Work out the finished part from the listing and answer in its coordinate system (mm). A direction names the side the tool comes from. Coordinates: 2 decimals unless noted, no trailing zeros. Order: outer loops, then holes, each group sorted by start corner. A loop starts at its lowest first (then second) coordinate and runs counter-clockwise, first axis right, second up. Notation, with made-up numbers: M 22,3 L 66,3 A16 cw 66,15 Z; hole C -11.5,38 d9. An arc over 180 degrees is marked long. Answer in a Markdown table with one row per item. Add a question column.
Item 1: Flat-ended cylindrical pins translate along their axes: pin 1 Ø3 at (x, z) = (1.5, 7) entering from -Y; pin 2 Ø1.1 at (x, y) = (2, 5) entering from +Z; pin 3 Ø5 at (x, z) = (-1, 112) entering from +Y; pin 4 Ø3 at (x, y) = (-3, 0) entering from -Z. Find the tip coordinate at first contact, or state that the pin passes through.
Item 2: Consider line 1 (X direction, y = 0, z = 7) (3 decimals); line 2 (Y direction, x = 0, z = 7.5) (3 decimals); line 3 (Y direction, x = 0.5, z = 112). Determine where each line is inside the solid, lowest interval first. Write a range as from..to.
Item 3: The part is cut by section D-D (z = 37). Write down the section's boundary in (x, y), then the cut area to 3 significant figures.
Item 4: The mould has two halves that part along X. Classify faces 5 (the face through (-1.38, -6.2, 62.61)), 6 (the face through (-2, 3, 0)), 7 (the face through (0, 0, 13.335)): released by +X, released by -X, zero draft, split by the parting line, or undercut.
Item 5: The part is cut by section A-A (y = 0). Write down the section's boundary in (x, z) (3 decimals), then the cut area to 3 significant figures.
Item 6: The part is cut by section B-B (x = 0). Write down the section's boundary in (y, z) (3 decimals).
Item 7: Which of the six approach directions +Z, -Z, +X, -X, +Y, -Y give full straight-line access (tool end or side, diameter ignored) to faces 1 (the face through (0, 5, 25.4)), 2 (the face through (-0.69, 3.1, 6.57)), 3 (the face through (0, -5, 25.4)), 4 (the face through (0, 4.191, 114))?
Item 8: The part is cut by section C-C (z = 19.5). Write down the section's boundary in (x, y), then the cut area to 3 significant figures.
from build123d import *

# Parameters (mm, degrees)
F0_R     = 6.35
F1_DEPTH = 127
F2_R     = 3.175
F3_DEPTH = 13.335
F4_R     = 3.175
F5_DEPTH = 13.335
F7_DEPTH = 25.4
F9_DEPTH = 25.4


with BuildPart() as f1:
    # F0 (on Top) → F1 (new body)
    with BuildSketch(Plane.XY):
        Circle(F0_R)
    extrude(amount=F1_DEPTH)

    # F2 (on face) → F3 (cut)
    with BuildSketch(Plane(origin=(0, 0, 0), x_dir=(1, 0, 0), z_dir=(0, 0, -1))):
        Circle(F2_R)
    extrude(amount=-F3_DEPTH, mode=Mode.SUBTRACT)

    # F4 (on face) → F5 (cut)
    with BuildSketch(Plane.XY.offset(127)):
        Circle(F4_R)
    extrude(amount=-F5_DEPTH, mode=Mode.SUBTRACT)

    # F6 (on face) → F7 (cut)
    with BuildSketch(Plane(origin=(0, 0, 0), x_dir=(1, 0, 0), z_dir=(0, 0, -1))):
        with BuildLine():
            Line((-4.7705365526, 4.191), (4.7705365526, 4.191))
            ThreePointArc((4.7705365526, 4.191), (0, 6.35), (-4.7705365526, 4.191))
        make_face()
        with BuildLine():
            Line((4.7705365526, -4.191), (-4.7705365526, -4.191))
            ThreePointArc((-4.7705365526, -4.191), (0, -6.35), (4.7705365526, -4.191))
        make_face()
    extrude(amount=-F7_DEPTH, mode=Mode.SUBTRACT)

    # F8 (on face) → F9 (cut)
    with BuildSketch(Plane.XY.offset(127)):
        with BuildLine():
            Line((4.7705365526, -4.191), (-4.7705365526, -4.191))
            ThreePointArc((-4.7705365526, -4.191), (0, -6.35), (4.7705365526, -4.191))
        make_face()
        with BuildLine():
            ThreePointArc((4.7705365526, 4.191), (0, 6.35), (-4.7705365526, 4.191))
            Line((-4.7705365526, 4.191), (4.7705365526, 4.191))
        make_face()
    extrude(amount=-F9_DEPTH, mode=Mode.SUBTRACT)


solid = f1.part
Reply:
| question | item | result |
|---|---|---|
| 1 | pin 1 | stops at y = -4.19 |
| 1 | pin 2 | stops at z = 101.6 |
| 1 | pin 3 | stops at y = 4.19 |
| 1 | pin 4 | stops at z = 0 |
| 2 | line 1 | x = -6.35..-3.175, 3.175..6.35 |
| 2 | line 2 | y = -4.191..-3.175, 3.175..4.191 |
| 2 | line 3 | y = -4.19..4.19 |
| 3 | outline | C 0,0 d12.7 |
| 3 | area | 127 mm2 |
| 4 | face 5 | split by the parting line |
| 4 | face 6 | zero draft |
| 4 | face 7 | undercut |
| 5 | outline | M -6.35,0 L -3.175,0 L -3.175,13.335 L 3.175,13.335 L 3.175,0 L 6.35,0 L 6.35,127 L 3.175,127 L 3.175,113.665 L -3.175,113.665 L -3.175,127 L -6.35,127 Z |
| 5 | area | 1,440 mm2 |
| 6 | outline | M -6.35,25.4 L -4.191,25.4 L -4.191,0 L -3.175,0 L -3.175,13.335 L 3.175,13.335 L 3.175,0 L 4.191,0 L 4.191,25.4 L 6.35,25.4 L 6.35,101.6 L 4.191,101.6 L 4.191,127 L 3.175,127 L 3.175,113.665 L -3.175,113.665 L -3.175,127 L -4.191,127 L -4.191,101.6 L -6.35,101.6 Z |
| 7 | face 1 | -Z, +X, -X, +Y |
| 7 | face 2 | -Z |
| 7 | face 3 | -Z, +X, -X, -Y |
| 7 | face 4 | +Z, +X, -X, +Y |
| 8 | outline | M -4.77,-4.19 L 4.77,-4.19 A6.35 ccw 4.77,4.19 L -4.77,4.19 A6.35 ccw Z |
| 8 | area | 98.1 mm2 |
